Study the drawing (mm; zero at the part's minimum x, y, z) and answer. A direction names the side the tool comes from. Give positions to 0.01 mm unless a question says otherwise; leave off trailing zeros. Order: outer loops, then holes, each group sorted by start corner. A loop starts at its lowest first (then second) coordinate and runs counter-clockwise, first axis right, second up.
Item 1: Find the intervals of material crossed by line 1 along Y through (x, z) = (3, 6); line 2 along X through (y, z) = (18.5, 0.75), in increasing order.
Item 2: The mould has two halves that part along Y. Classify the marked faces 3, 4 and 5: +Y half, -Y half, draft (parallel to the pull), parting line (faces both ways), or undercut.
Item 3: Which of the six approach directions +Z, -Z, +X, -X, +Y, -Y give full straight-line access (tool end or side, diameter ignored) to the marked faces 1 and 2?
Item 4: A cutting plane is placed at C-C (z = 3.5). Write down the section's boundary in (x, y).
Item 5: A cutting plane is placed at A-A (y = 13). Write down the section's boundary in (x, z).
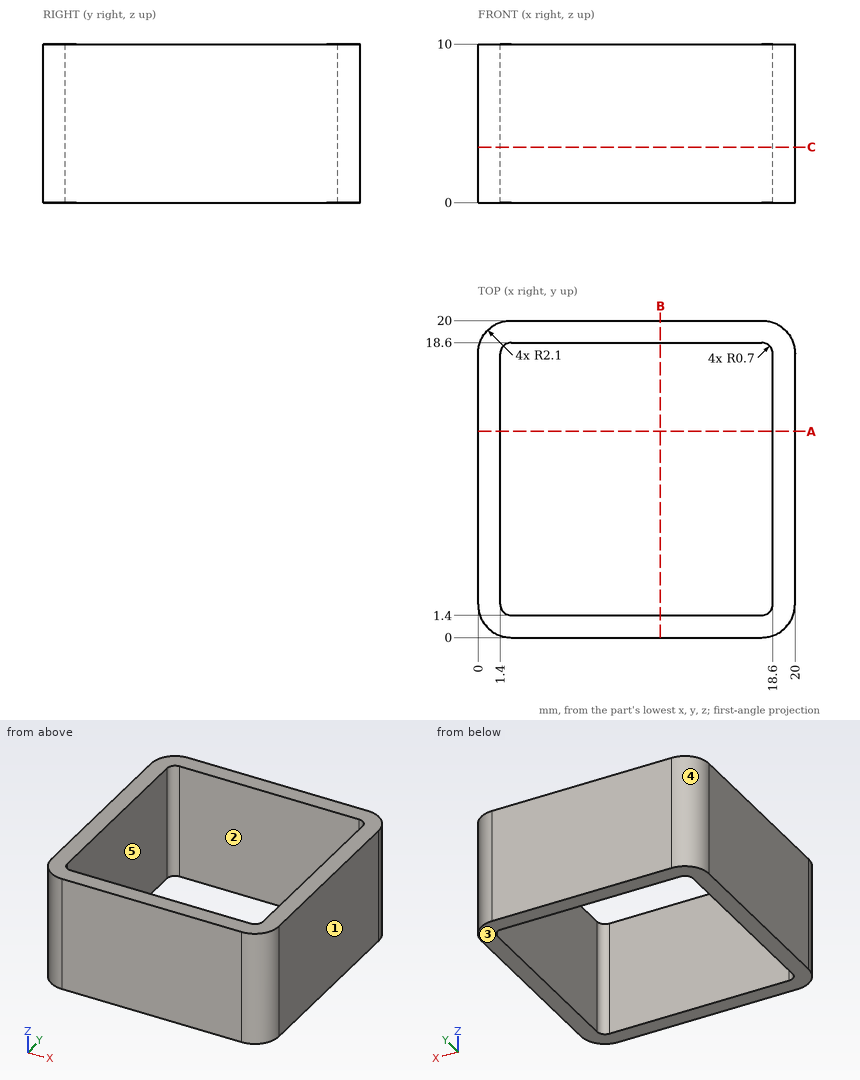
Response values:
1. line 1: y = 0 to 1.4, 18.6 to 20
1. line 2: x = 0.09 to 1.74, 18.26 to 19.91
2. face 3: draft
2. face 4: +Y half
2. face 5: undercut
3. face 1: +Z, -Z, +X, +Y, -Y
3. face 2: +Z, -Z
4. outline: (0, 2.1) arc R2.1 ccw to (2.1, 0) - (17.9, 0) arc R2.1 ccw to (20, 2.1) - (20, 17.9) arc R2.1 ccw to (17.9, 20) - (2.1, 20) arc R2.1 ccw to (0, 17.9) - close; hole (1.4, 2.1) arc R0.7 ccw to (2.1, 1.4) - (17.9, 1.4) arc R0.7 ccw to (18.6, 2.1) - (18.6, 17.9) arc R0.7 ccw to (17.9, 18.6) - (2.1, 18.6) arc R0.7 ccw to (1.4, 17.9) - close
5. outline: (0, 0) - (1.4, 0) - (1.4, 10) - (0, 10) - close; (18.6, 0) - (20, 0) - (20, 10) - (18.6, 10) - close
